```python
from build123d import *

# Parameters (mm, degrees)
SKETCH1_W                       = 100
SKETCH1_H                       = 50
BOSS_EXTRUDE1_DEPTH             = 5
SKETCH2_W                       = 5
SKETCH2_H                       = 50
BOSS_EXTRUDE2_DEPTH             = 22
SKETCH5_W                       = 25
SKETCH5_H                       = 4
BOSS_EXTRUDE3_DEPTH             = 16
SKETCH6_R                       = 1.25
HOLES_TO_FIX_LEVEL_SWITCH_DEPTH = 40
SKETCH10_W                      = 25
SKETCH10_H                      = 50
BOSS_EXTRUDE4_DEPTH             = 8
CUT_EXTRUDE2_DEPTH              = 61.074953184
CUT_EXTRUDE2_DEPTH_BACK         = 61.074953184
SKETCH9_W                       = 35
SKETCH9_H                       = 50
CUT_EXTRUDE3_DEPTH              = 10
SKETCH11_W                      = 27
SKETCH11_H                      = 50
CUT_EXTRUDE4_DEPTH              = 8


with BuildPart() as part:
    # Sketch1 → Boss-Extrude1 (new body)
    with BuildSketch(Plane.XY):
        Rectangle(SKETCH1_W, SKETCH1_H)
    extrude(amount=BOSS_EXTRUDE1_DEPTH)

    # Sketch2 → Boss-Extrude2 (add)
    with BuildSketch(Plane.XY):
        with Locations((22.5, 0)):
            Rectangle(SKETCH2_W, SKETCH2_H)
    extrude(amount=-BOSS_EXTRUDE2_DEPTH)

    # Sketch5 → Boss-Extrude3 (add)
    with BuildSketch(Plane.XY):
        with Locations((2.5, 17)):
            Rectangle(SKETCH5_W, SKETCH5_H)
    extrude(amount=-BOSS_EXTRUDE3_DEPTH)

    # Sketch6 → Holes-to-fix-level-switch (cut)
    with BuildSketch(Plane(origin=(0, 19, 0), x_dir=(1, 0, 0), z_dir=(0, 1, 0))):
        with Locations(Location((-4.68, 10, 0), (0, 0, 270))):
            Circle(SKETCH6_R)
        with Locations(Location((4.04, 10, 0), (0, 0, 270))):
            Circle(SKETCH6_R)
    extrude(amount=-HOLES_TO_FIX_LEVEL_SWITCH_DEPTH, mode=Mode.SUBTRACT)

    # Sketch10 → Boss-Extrude4 (add)
    with BuildSketch(Plane(origin=(0, 0, 0), x_dir=(-1, 0, 0), z_dir=(0, 0, -1))):
        with Locations((-37.5, 0)):
            Rectangle(SKETCH10_W, SKETCH10_H)
    extrude(amount=BOSS_EXTRUDE4_DEPTH)

    # Sketch8 → Cut-Extrude2 (cut, two sides: drawn at the far end of the back side and taken through both)
    with BuildSketch(Plane.XY.offset(-CUT_EXTRUDE2_DEPTH_BACK)):
        with BuildLine():
            Line((33, 16.75), (43, 16.75))
            ThreePointArc((43, 16.75), (44.75, 15), (43, 13.25))
            Line((43, 13.25), (33, 13.25))
            ThreePointArc((33, 13.25), (31.25, 15), (33, 16.75))
        make_face()
        with BuildLine():
            Line((33, -13.25), (43, -13.25))
            ThreePointArc((43, -13.25), (44.75, -15), (43, -16.75))
            Line((43, -16.75), (33, -16.75))
            ThreePointArc((33, -16.75), (31.25, -15), (33, -13.25))
        make_face()
    extrude(amount=CUT_EXTRUDE2_DEPTH + CUT_EXTRUDE2_DEPTH_BACK, mode=Mode.SUBTRACT)

    # Sketch9 → Cut-Extrude3 (cut)
    with BuildSketch(Plane(origin=(0, 0, 0), x_dir=(-1, 0, 0), z_dir=(0, 0, -1))):
        with Locations((32.5, 0)):
            Rectangle(SKETCH9_W, SKETCH9_H)
    extrude(amount=-CUT_EXTRUDE3_DEPTH, mode=Mode.SUBTRACT)

    # Sketch11 → Cut-Extrude4 (cut)
    with BuildSketch(Plane.XY.offset(5)):
        with Locations((36.5, 0)):
            Rectangle(SKETCH11_W, SKETCH11_H)
    extrude(amount=-CUT_EXTRUDE4_DEPTH, mode=Mode.SUBTRACT)


solid = part.part
```
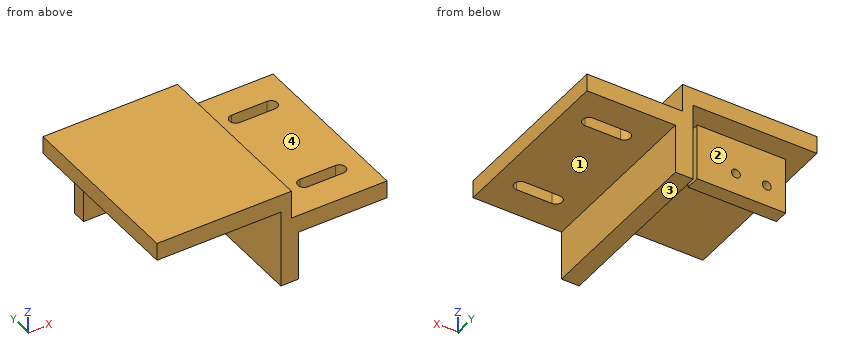
Geometry check sheet. Reference: the model listing, model coordinates, mm. Face numbers are marked on the shaded views. A direction names the side the tool comes from. Coordinates: 2 decimals unless noted, no trailing zeros. Write each loop counter-clockwise with the first axis right and the second up, starting at its lowest first coordinate (ties: lowest second). Pieces come first, ordered by that corner, then holes. Notation, with made-up numbers: (67.5, -37.5) -> (102.5, -37.5) arc R13 cw to (102.5, -18.5) -> close; hole circle Ø2 at (-28, -31.75). An arc over 180 degrees is marked (long way). Use CSV: the item, a comma, the result in double quotes. Start each with the question number.
Item 1: Cross-section at D-D, the plane z = -12. Record the cut outline in (x, y), plus the area to 3 significant figures.
Item 2: Cross-section at C-C, the plane y = -15. Record the cut outline in (x, z).
Item 3: Cross-section at B-B, the plane x = 39. Record the cut outline in (y, z), plus the area to 3 significant figures.
Item 4: Depth check by flat-ended pin: pin 1 Ø8 at (x, z) = (-1, -12) entering from +Y; pin 2 Ø11 at (y, z) = (-4, -15.5) entering from -X; pin 3 Ø17.5 at (x, y) = (-6, 7) entering from -Z. Enter the tip coordinate at first touch or a pass-through.
Item 5: Set-up check for the marked faces 1, 2, 3 and 4: record each of +Z, -Z, +X, -X, +Y, -Y from which the full face is reachable in a straight line by a thin tool's end or side.
Item 6: Cross-section at A-A, the plane z = -7. Record the cut outline in (x, y), plus the area to 3 significant figures.
Item 7: Thickness scan on line 1 (X direction, y = 16.6, z = -10); line 2 (Y direction, x = 39, z = -5.25); line 3 (Y direction, x = 11, z = -8.5). Record the ranges inside material, lowest first.
Answers:
1,outline,"(-10, 15) -> (15, 15) -> (15, 19) -> (-10, 19) -> close; (20, -25) -> (25, -25) -> (25, 25) -> (20, 25) -> close"
1,area,"350 mm^2"
2,outline,"(-15, 0) -> (20, 0) -> (20, -22) -> (25, -22) -> (25, -8) -> (31.25, -8) -> (31.25, -3) -> (23, -3) -> (23, 5) -> (-15, 5) -> close; (44.75, -8) -> (50, -8) -> (50, -3) -> (44.75, -3) -> close"
3,outline,"(-25, -8) -> (-16.75, -8) -> (-16.75, -3) -> (-25, -3) -> close; (-13.25, -8) -> (13.25, -8) -> (13.25, -3) -> (-13.25, -3) -> close; (16.75, -8) -> (25, -8) -> (25, -3) -> (16.75, -3) -> close"
3,area,"215 mm^2"
4,pin 1,"y = 19"
4,pin 2,"x = 20"
4,pin 3,"z = -16"
5,face 1,"-Z, +X, +Y, -Y"
5,face 2,"-Z, -X, +Y"
5,face 3,"-Z, +X, -X, +Y, -Y"
5,face 4,"+Z, +X, +Y, -Y"
6,outline,"(-10, 15) -> (15, 15) -> (15, 19) -> (-10, 19) -> close; (20, -25) -> (50, -25) -> (50, 25) -> (20, 25) -> close; hole (33, -16.75) -> (43, -16.75) arc R1.75 ccw to (43, -13.25) -> (33, -13.25) arc R1.75 ccw to start; hole (33, 13.25) -> (43, 13.25) arc R1.75 ccw to (43, 16.75) -> (33, 16.75) arc R1.75 ccw to start"
6,area,"1,510 mm^2"
7,line 1,"-10 to -5.93, -3.43 to 2.79, 5.29 to 15, 20 to 25"
7,line 2,"-25 to -16.75, -13.25 to 13.25, 16.75 to 25"
7,line 3,"15 to 19"
